from build123d import *

# Parameters (mm, degrees)
BOSS_EXTRUDE1_DEPTH = 20
SKETCH2_W           = 36
SKETCH2_H           = 43
SKETCH2_W_2         = 68
SKETCH2_H_2         = 22
CUT_EXTRUDE1_DEPTH  = 17
SKETCH3_W           = 36
SKETCH3_H           = 9.142135624
CUT_EXTRUDE2_DEPTH  = 8
CUT_EXTRUDE3_REACH  = 102.441


with BuildPart() as part:
    # Sketch1 → Boss-Extrude1 (new body)
    with BuildSketch(Plane(origin=(0, 0, 0), x_dir=(1, 0, 0), z_dir=(0, 1, 0))):
        Polygon((-35, 43.142135624), (35, 43.142135624), (49.142135624, 29), (49.142135624, -29), (35, -43.142135624), (-35, -43.142135624), (-49.142135624, -29), (-49.142135624, 29), align=None)
    extrude(amount=BOSS_EXTRUDE1_DEPTH)

    # Sketch2 → Cut-Extrude1 (cut)
    with BuildSketch(Plane(origin=(0, 20, 0), x_dir=(1, 0, 0), z_dir=(0, 1, 0))):
        with Locations((0, 20.642135624)):
            Rectangle(SKETCH2_W, SKETCH2_H)
        with Locations((0, -21)):
            Rectangle(SKETCH2_W_2, SKETCH2_H_2)
    extrude(amount=-CUT_EXTRUDE1_DEPTH, mode=Mode.SUBTRACT)

    # Sketch3 → Cut-Extrude2 (cut)
    with BuildSketch(Plane(origin=(0, 20, 0), x_dir=(1, 0, 0), z_dir=(0, 1, 0))):
        with Locations((0, -5.428932188)):
            Rectangle(SKETCH3_W, SKETCH3_H)
    extrude(amount=-CUT_EXTRUDE2_DEPTH, mode=Mode.SUBTRACT)

    # Sketch4 → Cut-Extrude3 (cut, up to next)
    with BuildSketch(Plane.XY.offset(-42.142135624), mode=Mode.PRIVATE) as cut_extrude3_sk1:
        with BuildLine():
            Line((-10.2, 10.13), (-5.2, 10.13))
            ThreePointArc((-5.2, 10.13), (-3.2, 8.13), (-5.2, 6.13))
            Line((-5.2, 6.13), (-10.2, 6.13))
            ThreePointArc((-10.2, 6.13), (-12.2, 8.13), (-10.2, 10.13))
        make_face()
    cut_extrude3_tool1 = extrude(cut_extrude3_sk1.sketch, amount=-CUT_EXTRUDE3_REACH, mode=Mode.PRIVATE) & part.part
    add(cut_extrude3_tool1.solids().sort_by_distance((-7.7, 8.13, -42.142136))[0], mode=Mode.SUBTRACT)


solid = part.part
Can you work these out from the model? Positions are in its coordinate system, mm. A direction names the side the tool comes from. Round coordinates to 2 decimals unless told otherwise and drop trailing zeros. Loops run counter-clockwise (first coordinate to the right, second up) from the corner with the lowest first, then second, coordinate; pieces in that order, holes last. Notation, with made-up numbers: (-16, 75) - (7, 75) arc R15 cw to (7, 80) - close; hole circle Ø10 at (-15.5, 11). An arc over 180 degrees is marked (long way). Answer in a Markdown table with one row per item. Add a question column.
Q1. I want a section at C-C on x = 15.5. List the corners of the cut face in (y, z) for me.
Q2. I want a section at D-D on z = 2.5. List the corners of the cut face in (x, y) for me, and give its area (3 significant figures).
Q3. I need wall thicknesses on L1, parallel to Z at x = 16.5, y = 6; L2, parallel to X at y = 14.75, z = 20.5; L3, parallel to X at y = 19, z = 2.5. Which ranges of each line are inside material? Lowest first, please.
Q4. I want a section at B-B on y = 4.75. List the corners of the cut face in (x, z) for me, and give its area (3 significant figures).
Q5. We'd pull the mould along Z, two halves only. Please class faces 3 (the flat face through (42.17, 9.86, 35.97)), 4 (the flat face through (-49.142, 10, 0)), 5 (the flat face through (-42.17, 9.86, -35.97)), 6 (the flat face through (0, 8, 0.858)): pulls with the +Z half, pulls with the -Z half, needs draft (parallel to the pull), parting line crosses it, or undercut.
Q6. For pin 1 Ø11 at (x, z) = (-4.5, 23.5) entering from +Y; pin 2 Ø4 at (y, z) = (8, 32.5) entering from +X; pin 3 Ø7.5 at (x, z) = (7, 6) entering from +Y, each with a flat end and sliding along its axis, tell me the tip position at first contact or that it passes through.
Q7. Which directions (+Z, -Z, +X, -X, +Y, -Y) give clear straight access to the entire face, cutting with the end or side of a thin tool? Please do faces 1 (the flat face through (0, 10, -43.142)), 2 (the flat face through (0, 12, -42.142)).
Q8. I want a section at A-A on y = 18. List the corners of the cut face in (x, z) for me, and give its area (3 significant figures).
A:
| question | item | result |
|---|---|---|
| 1 | outline | (0, -43.14) - (20, -43.14) - (20, -42.14) - (3, -42.14) - (3, 0.86) - (12, 0.86) - (12, 10) - (3, 10) - (3, 32) - (20, 32) - (20, 43.14) - (0, 43.14) - close |
| 2 | outline | (-49.14, 0) - (49.14, 0) - (49.14, 20) - (18, 20) - (18, 12) - (-18, 12) - (-18, 20) - (-49.14, 20) - close |
| 2 | area | 1,680 mm^2 |
| 3 | L1 | -43.14 to -42.14, 0.86 to 10, 32 to 43.14 |
| 3 | L2 | -49.14 to -34, 34 to 49.14 |
| 3 | L3 | -49.14 to -18, 18 to 49.14 |
| 4 | outline | (-49.14, -29) - (-35, -43.14) - (35, -43.14) - (49.14, -29) - (49.14, 29) - (35, 43.14) - (-35, 43.14) - (-49.14, 29) - close; hole (-34, 10) - (34, 10) - (34, 32) - (-34, 32) - close; hole (-18, -42.14) - (18, -42.14) - (18, 0.86) - (-18, 0.86) - close |
| 4 | area | 5,040 mm^2 |
| 5 | face 3 | pulls with the +Z half |
| 5 | face 4 | needs draft |
| 5 | face 5 | pulls with the -Z half |
| 5 | face 6 | undercut |
| 6 | pin 1 | y = 3 |
| 6 | pin 2 | x = 47.64 |
| 6 | pin 3 | y = 12 |
| 7 | face 1 | -Z, +X, -X, +Y, -Y |
| 7 | face 2 | +Y |
| 8 | outline | (-49.14, -29) - (-35, -43.14) - (35, -43.14) - (49.14, -29) - (49.14, 29) - (35, 43.14) - (-35, 43.14) - (-49.14, 29) - close; hole (-34, 10) - (-18, 10) - (-18, -42.14) - (18, -42.14) - (18, 10) - (34, 10) - (34, 32) - (-34, 32) - close |
| 8 | area | 4,710 mm^2 |
